Part model, mm, in its own coordinate system. Face numbers are marked on the shaded views. Give positions to 0.01 mm unless a question says otherwise; leave off trailing zeros. Order: outer loops, then holes, each group sorted by start corner. A loop starts at its lowest first (then second) coordinate and runs counter-clockwise, first axis right, second up. Notation, with made-up numbers: (54.5, -40) -> (66.5, -40) arc R30 ccw to (66.5, -15) -> close; hole circle Ø10 at (38.5, 45). An arc over 180 degrees is marked (long way). Write item = value, one per line. Start each with the question number.
Item 1: Band-saw the part on C-C on z = -26.25. Count the separate pieces of the cut face and the enclosed holes in it, plus the area to 3 significant figures.
Item 2: Flat gauge pins, fed straight in: P1, Ø2.5, axis at x = -17.22, y = 41.57, coming from the -Z side; P2, Ø1, axis at y = -23.5, z = -27, coming from the +X side; P3, Ø1.5, axis at y = 13, z = -23.5, coming from the +X side. Where does each tip first touch, or does it go through?
Item 3: Drill centre lines: line 1 along X through (y, z) = (-16.5, -24.25); line 2 along Y through (x, z) = (-4, -29.5); line 3 along X through (y, z) = (-14.5, -26.5). Where is each one in solid material? Low to high.
Item 4: Band-saw the part on A-A on y = 0. Write the cut outline in (x, z).
Item 5: Pull direction X, two halves, no side cores. Call the marked faces 1, 2 and 3: +X half, -X half, draft (parallel to the pull), parting line (faces both ways), or undercut.
```python
from build123d import *

# Parameters (mm, degrees)
CYLINDER662_R               = 1.5
CYLINDER662_DEPTH           = 20
CYLINDER662_PLACEMENT_ANGLE = 45
CYLINDER664_R               = 1.5
CYLINDER664_DEPTH           = 20
CYLINDER661_R               = 1.5
CYLINDER661_DEPTH           = 20
CYLINDER661_PLACEMENT_ANGLE = 135
CYLINDER663_R               = 1.5
CYLINDER663_DEPTH           = 20
CYLINDER667_R               = 1.5
CYLINDER667_DEPTH           = 20
CYLINDER667_PLACEMENT_ANGLE = 225
CYLINDER665_R               = 1.5
CYLINDER665_DEPTH           = 20
CYLINDER666_R               = 1.5
CYLINDER666_DEPTH           = 20
CYLINDER666_PLACEMENT_ANGLE = 45
CYLINDER660_R               = 1.5
CYLINDER660_DEPTH           = 20
COMPOUND661_PLACEMENT_ANGLE = 22.5
TUBE041_R                   = 49
TUBE041_R_2                 = 42
TUBE041_DEPTH               = 10


with BuildPart() as obj1:
    # Cylinder662 → Cylinder662 (new body)
    with BuildSketch(Plane.XY):
        Circle(CYLINDER662_R)
    extrude(amount=CYLINDER662_DEPTH)


with BuildPart() as obj1_1:
    # Cylinder662 placement: moved
    add(obj1.part.moved(Location((-31.819805, 31.819805, -18))).rotate(Axis((-31.819805, 31.819805, -18), (0, 0, 1)), CYLINDER662_PLACEMENT_ANGLE))


with BuildPart() as obj2:
    # Cylinder664 → Cylinder664 (new body)
    with BuildSketch(Plane(origin=(-45, 0, -18), x_dir=(0, 1, 0), z_dir=(0, 0, 1))):
        Circle(CYLINDER664_R)
    extrude(amount=CYLINDER664_DEPTH)


with BuildPart() as obj3:
    # Cylinder661 → Cylinder661 (new body)
    with BuildSketch(Plane.XY):
        Circle(CYLINDER661_R)
    extrude(amount=CYLINDER661_DEPTH)


with BuildPart() as obj3_1:
    # Cylinder661 placement: moved
    add(obj3.part.moved(Location((-31.819805, -31.819805, -18))).rotate(Axis((-31.819805, -31.819805, -18), (0, 0, 1)), CYLINDER661_PLACEMENT_ANGLE))


with BuildPart() as obj4:
    # Cylinder663 → Cylinder663 (new body)
    with BuildSketch(Plane(origin=(0, -45, -18), x_dir=(-1, 0, 0), z_dir=(0, 0, 1))):
        Circle(CYLINDER663_R)
    extrude(amount=CYLINDER663_DEPTH)


with BuildPart() as obj5:
    # Cylinder667 → Cylinder667 (new body)
    with BuildSketch(Plane.XY):
        Circle(CYLINDER667_R)
    extrude(amount=CYLINDER667_DEPTH)


with BuildPart() as obj5_1:
    # Cylinder667 placement: moved
    add(obj5.part.moved(Location((31.819805, -31.819805, -18))).rotate(Axis((31.819805, -31.819805, -18), (0, 0, 1)), CYLINDER667_PLACEMENT_ANGLE))


with BuildPart() as obj6:
    # Cylinder665 → Cylinder665 (new body)
    with BuildSketch(Plane(origin=(45, 0, -18), x_dir=(0, -1, 0), z_dir=(0, 0, 1))):
        Circle(CYLINDER665_R)
    extrude(amount=CYLINDER665_DEPTH)


with BuildPart() as obj7:
    # Cylinder666 → Cylinder666 (new body)
    with BuildSketch(Plane.XY):
        Circle(CYLINDER666_R)
    extrude(amount=CYLINDER666_DEPTH)


with BuildPart() as obj7_1:
    # Cylinder666 placement: moved
    add(obj7.part.moved(Location((31.819805, 31.819805, -18))).rotate(Axis((31.819805, 31.819805, -18), (0, 0, -1)), CYLINDER666_PLACEMENT_ANGLE))


with BuildPart() as compound661:
    # Cylinder660 → Cylinder660 (new body)
    with BuildSketch(Plane(origin=(0, 45, -18), x_dir=(1, 0, 0), z_dir=(0, 0, 1))):
        Circle(CYLINDER660_R)
    extrude(amount=CYLINDER660_DEPTH)

    # Compound661: union obj1, obj2, obj3, obj4, obj5, obj6, obj7
    add(obj1_1.part)
    add(obj2.part)
    add(obj3_1.part)
    add(obj4.part)
    add(obj5_1.part)
    add(obj6.part)
    add(obj7_1.part)


with BuildPart() as compound661_1:
    # Compound661 placement: moved
    add(compound661.part.moved(Location((0, 0, -8))).rotate(Axis((0, 0, -8), (0, 0, 1)), COMPOUND661_PLACEMENT_ANGLE))


with BuildPart() as cut291:
    # Tube041 → Tube041 (new body)
    with BuildSketch(Plane.XY.offset(-22)):
        Circle(TUBE041_R)
        Circle(TUBE041_R_2, mode=Mode.SUBTRACT)
    extrude(amount=TUBE041_DEPTH)

    # Cut291: cut Compound661
    add(compound661_1.part, mode=Mode.SUBTRACT)


with BuildPart() as cut291_1:
    # Cut291 placement: moved
    add(cut291.part.moved(Location((0, 0, -10))))


solid = cut291_1.part
```
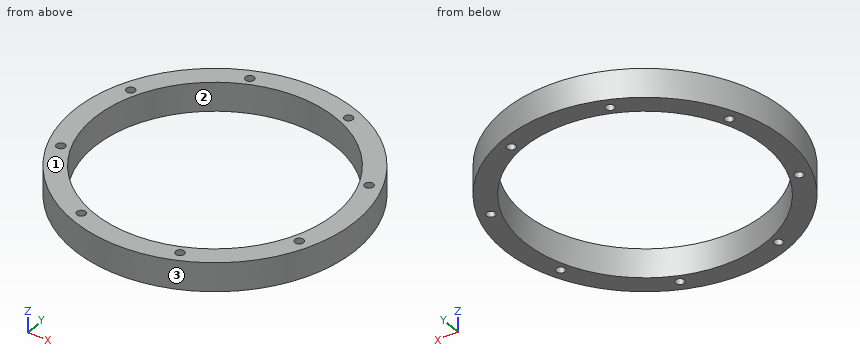
Values found:
q1.separate_pieces = 1
q1.enclosed_holes = 9
q1.area = 1,940 mm^2
q2.P1 = through
q2.P2 = 43.27
q2.P3 = 47.44
q3.line_1 = -46.14 to -42.89, -40.26 to -38.62, 38.62 to 40.26, 42.89 to 46.14
q3.line_2 = -48.84 to -41.81, 41.81 to 48.84
q3.line_3 = -46.81 to -39.42, 39.42 to 46.81
q4.outline = (-49, -32) -> (-42, -32) -> (-42, -22) -> (-49, -22) -> close; (42, -32) -> (49, -32) -> (49, -22) -> (42, -22) -> close
q5.face_1 = draft
q5.face_2 = undercut
q5.face_3 = parting line
